Build history of the part. All positions in model axes, mm. A direction names the side the tool comes from. Round coordinates to 2 decimals unless told otherwise and drop trailing zeros. Write each loop counter-clockwise with the first axis right and the second up, starting at its lowest first coordinate (ties: lowest second). Pieces come first, ordered by that corner, then holes. Notation, with made-up numbers: (51.25, 53.25) -> (78.25, 53.25) arc R16 cw to (78.25, 64.25) -> close; hole circle Ø6 at (-32, 54). An arc over 180 degrees is marked (long way). Answer in a Markdown table with one row per item.
```python
from build123d import *

# Parameters (mm, degrees)
F0_W     = 20.32
F0_H     = 12.7
F1_DEPTH = 3.175
F2_W     = 20.32
F2_H     = 3.175
F3_DEPTH = 14.605
F4_R     = 8.255
F5_DEPTH = 17.78
F6_W     = 20.32
F6_H     = 17.78
F7_DEPTH = 3.175
F8_W     = 3.386666
F8_H     = 3.386666
F9_DEPTH = 15.24


with BuildPart() as f1:
    # F0 (on Top) → F1 (new body)
    with BuildSketch(Plane.XY):
        Rectangle(F0_W, F0_H)
    extrude(amount=F1_DEPTH)

    # F2 (on face) → F3 (join)
    with BuildSketch(Plane.XY.offset(3.175)):
        with Locations((0, -4.7625)):
            Rectangle(F2_W, F2_H)
    extrude(amount=F3_DEPTH)

    # F4 (on Top) → F5 (join)
    with BuildSketch(Plane.XY):
        with BuildLine():
            Line((10.16, 3.175), (10.16, 14.605))
            ThreePointArc((10.16, 14.605), (0, 24.765), (-10.16, 14.605))
            Line((-10.16, 14.605), (-10.16, 3.175))
            Line((-10.16, 3.175), (10.16, 3.175))
        make_face()
        with Locations((0, 14.605)):
            Circle(F4_R, mode=Mode.SUBTRACT)
    extrude(amount=F5_DEPTH)

    # F6 (on face) → F7 (join)
    with BuildSketch(Plane.XZ.offset(6.35)):
        with Locations((0, 8.89)):
            Rectangle(F6_W, F6_H)
    extrude(amount=F7_DEPTH)

    # F8 (on face) → F9 (cut)
    with BuildSketch(Plane.XZ.offset(9.525)):
        with Locations((-5.08, 8.89)):
            Rectangle(F8_W, F8_H)
        with Locations((5.08, 8.89)):
            Rectangle(F8_W, F8_H)
    extrude(amount=-F9_DEPTH, mode=Mode.SUBTRACT)


solid = f1.part
```
Q1. Saw through at D-D on x = -5.5. Write the cut outline in (y, z) (3 decimals), plus the area to 3 significant figures.
A:
| item | result |
|---|---|
| outline | (-9.525, 0) -> (8.449, 0) -> (8.449, 17.78) -> (3.175, 17.78) -> (3.175, 10.583) -> (5.715, 10.583) -> (5.715, 7.197) -> (3.175, 7.197) -> (3.175, 3.175) -> (-3.175, 3.175) -> (-3.175, 7.197) -> (-9.525, 7.197) -> close; (-9.525, 10.583) -> (-3.175, 10.583) -> (-3.175, 17.78) -> (-9.525, 17.78) -> close; (20.761, 0) -> (23.148, 0) -> (23.148, 17.78) -> (20.761, 17.78) -> close |
| area | 239 mm² |
Q2. Saw through at A-A on x = 0. Write the cut outline in (y, z) (3 decimals).
A:
| item | result |
|---|---|
| outline | (-9.525, 0) -> (6.35, 0) -> (6.35, 17.78) -> (3.175, 17.78) -> (3.175, 3.175) -> (-3.175, 3.175) -> (-3.175, 17.78) -> (-9.525, 17.78) -> close; (22.86, 0) -> (24.765, 0) -> (24.765, 17.78) -> (22.86, 17.78) -> close |
Q3. Drop flat-ended pins along their axis: P1, Ø3, axis at y = 20, z = 8, coming from the -X side; P2, Ø1.9, axis at x = 0, y = 0, coming from the +Z side (3 decimals); P3, Ø1.7, axis at x = -4.5, z = 9.5, coming from the -Y side (3 decimals); P4, Ø1.5, axis at x = -5, y = 18.5, coming from the +Z side. Give the stop position or say it passes through.
A:
| item | result |
|---|---|
| P1 | x = -9.38 |
| P2 | z = 3.175 |
| P3 | y = 5.715 |
| P4 | through |
Q4. Two-plate mould, pull along Z, no slides. Class faces 1 (the flat face through (10.16, 5, 9)), 2 (the flat face through (5, 4, 10.583)), 3 (the flat face through (4, 7, 17.78)): released by +Z, released by -Z, zero draft, split by the parting line, or undercut.
A:
| item | result |
|---|---|
| face 1 | zero draft |
| face 2 | undercut |
| face 3 | released by +Z |
Q5. Saw through at B-B on z = 9.75. Write the cut outline in (x, y) (3 decimals), plus the area to 3 significant figures.
A:
| item | result |
|---|---|
| outline | (-10.16, -9.525) -> (-6.773, -9.525) -> (-6.773, -3.175) -> (-10.16, -3.175) -> close; (-10.16, 3.175) -> (-6.773, 3.175) -> (-6.773, 5.715) -> (-3.387, 5.715) -> (-3.387, 3.175) -> (3.387, 3.175) -> (3.387, 5.715) -> (6.773, 5.715) -> (6.773, 3.175) -> (10.16, 3.175) -> (10.16, 14.605) arc R10.16 ccw to (-10.16, 14.605) -> close; (-3.387, -9.525) -> (3.387, -9.525) -> (3.387, -3.175) -> (-3.387, -3.175) -> close; (6.773, -9.525) -> (10.16, -9.525) -> (10.16, -3.175) -> (6.773, -3.175) -> close; hole circle Ø16.51 at (0, 14.605) |
| area | 249 mm² |
Q6. Saw through at C-C on y = -5.5. Write the cut outline in (x, z), plus the area to 3 significant figures.
A:
| item | result |
|---|---|
| outline | (-10.16, 0) -> (10.16, 0) -> (10.16, 17.78) -> (-10.16, 17.78) -> close; hole (-6.77, 7.2) -> (-3.39, 7.2) -> (-3.39, 10.58) -> (-6.77, 10.58) -> close; hole (3.39, 7.2) -> (6.77, 7.2) -> (6.77, 10.58) -> (3.39, 10.58) -> close |
| area | 338 mm² |
Q7. Which spindle directions (+Z, -Z, +X, -X, +Y, -Y) get a long thin tool onto all of the face, cutting with end or side? Do faces 4 (the flat face through (5, -6, 10.583)), 5 (the cylindrical face through (0.223, 24.763, 8.766)), 6 (the flat face through (0, 3.175, 10)). Say none if no direction does.
A:
| item | result |
|---|---|
| face 4 | -Y |
| face 5 | +Z, -Z, +Y |
| face 6 | +Z, +X, -X |
Q8. Wall check: line 1 (Y direction, x = 0, z = 8.25) (3 decimals); line 2 (Y direction, x = 7.25, z = 13.5) (3 decimals); line 3 (X direction, y = -4.5, z = 10). Give the ranges that are in metal, low to high. Write a range as [from, to].
A:
| item | result |
|---|---|
| line 1 | [-9.525, -3.175], [3.175, 6.35], [22.86, 24.765] |
| line 2 | [-9.525, -3.175], [3.175, 10.658], [18.552, 21.723] |
| line 3 | [-10.16, -6.77], [-3.39, 3.39], [6.77, 10.16] |
